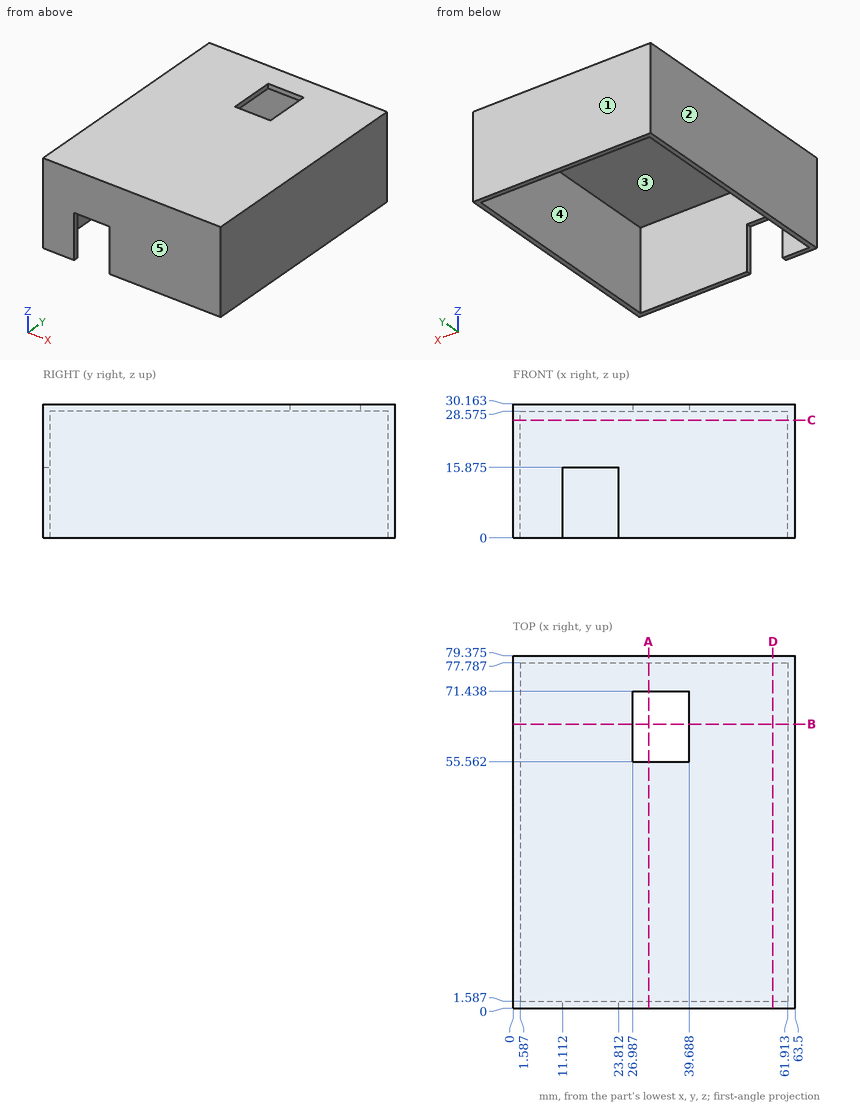
Verification items for this drawing (mm, ordinates from the low corner). A direction names the side the tool comes from. Coordinates: 2 decimals unless noted, no trailing zeros. Loops run counter-clockwise (first coordinate to the right, second up) from the corner with the lowest first, then second, coordinate; pieces in that order, holes last. Notation, with made-up numbers: (57, 36) -> (112, 36) arc R32 ccw to (112, 71) -> close; hole circle Ø3 at (2, 67.25). An arc over 180 degrees is marked (long way). Answer in a Markdown table with one row per item. Add a question column.
1. Section check C-C, the plane z = 26.5. Enter the section's corners in (x, y) (1 decimal).
2. Material ranges on probe 1 along X at (y, z) = (60, 23); probe 2 along Y at (x, z) = (35.5, 27.5) (1 decimal); probe 3 along Z at (x, y) = (14, 42) (1 decimal), recorded low to high. Write a range as [from, to].
3. Depth check by flat-ended pin: P1, Ø5, axis at y = 21, z = 15.5, coming from the -X side; P2, Ø5, axis at x = 54.5, y = 38.5, coming from the -Z side (1 decimal); P3, Ø0.5, axis at x = 20.5, y = 1, coming from the -Z side (1 decimal). Enter the tip coordinate at first touch or a pass-through.
4. Section check D-D, the plane x = 58.5. Enter the section's corners in (y, z) (1 decimal).
5. Access from +Z, -Z, +X, -X, +Y, -Y to the whole of each face (thin tool, end or side, straight path). Record for the marked faces 4 and 5.
6. Section check A-A, the plane x = 30.5. Enter the section's corners in (y, z) (1 decimal).
7. Section check B-B, the plane y = 64. Enter the section's corners in (x, z) (1 decimal).
8. Draft check along Y on the marked faces 1, 2 and 3. Enter one of: +Y half, -Y half, draft (parallel to the pull), parting line (faces both ways), or undercut.
Derived:
| question | item | result |
|---|---|---|
| 1 | outline | (0, 0) -> (63.5, 0) -> (63.5, 79.4) -> (0, 79.4) -> close; hole (1.6, 1.6) -> (61.9, 1.6) -> (61.9, 77.8) -> (1.6, 77.8) -> close |
| 2 | probe 1 | x = [0, 1.59], [61.91, 63.5] |
| 2 | probe 2 | y = [0, 1.6], [77.8, 79.4] |
| 2 | probe 3 | z = [28.6, 30.2] |
| 3 | P1 | stops at x = 0 |
| 3 | P2 | stops at z = 28.6 |
| 3 | P3 | stops at z = 15.9 |
| 4 | outline | (0, 0) -> (1.6, 0) -> (1.6, 28.6) -> (77.8, 28.6) -> (77.8, 0) -> (79.4, 0) -> (79.4, 30.2) -> (0, 30.2) -> close |
| 5 | face 4 | -Z |
| 5 | face 5 | +Z, -Z, +X, -X, -Y |
| 6 | outline | (0, 0) -> (1.6, 0) -> (1.6, 28.6) -> (55.6, 28.6) -> (55.6, 30.2) -> (0, 30.2) -> close; (71.4, 28.6) -> (77.8, 28.6) -> (77.8, 0) -> (79.4, 0) -> (79.4, 30.2) -> (71.4, 30.2) -> close |
| 7 | outline | (0, 0) -> (1.6, 0) -> (1.6, 28.6) -> (27, 28.6) -> (27, 30.2) -> (0, 30.2) -> close; (39.7, 28.6) -> (61.9, 28.6) -> (61.9, 0) -> (63.5, 0) -> (63.5, 30.2) -> (39.7, 30.2) -> close |
| 8 | face 1 | +Y half |
| 8 | face 2 | draft |
| 8 | face 3 | undercut |
